For this review, use the dimensioned drawing (mm, ordinates from the lowest corner) and the shaded views. A direction names the side the tool comes from. Round coordinates to 2 decimals unless told otherwise and drop trailing zeros. Loops run counter-clockwise (first coordinate to the right, second up) from the corner with the lowest first, then second, coordinate; pieces in that order, holes last. Notation, with made-up numbers: (51.25, 47) - (74.25, 47) arc R10 cw to (74.25, 53) - close; hole circle Ø11 at (-40, -15). An arc over 180 degrees is marked (long way). Use one line per item in the form item = value. Start each with the question number.
(1) We need section B-B, the plane y = 5.25. Write out the cut boundary in (x, z).
(2) Machinability: for the marked faces 4, 5 and 6, which of the approach directions +Z, -Z, +X, -X, +Y, -Y give a long, thin tool a straight path to every point of the face, cutting with its end or side? Answer none if there is none.
(3) The part is to be moulded in two halves that separate along Z. For the marked faces 1, 2 and 3, say which applies: released by +Z, released by -Z, zero draft, split by the parting line, or undercut.
(4) Wall thickness on probe 1 along X at (y, z) = (0.75, 4.5); probe 2 along Z at (x, y) = (5.75, 3.25); probe 3 along Z at (x, y) = (3.75, 1): over which ranges is each line inside the solid? List them lowest first. Write a range as [from, to].
(5) We need section A-A, the plane x = 5.25. Write out the cut boundary in (y, z).
(6) For pin 1 (1.5 mm diameter, centred on x = 4.5, y = 2, fed in from -Z); pin 2 (1.5 mm diameter, centred on x = 4.5, z = 1.5, fed in from +Y), all flat-tipped, find the tip position at first contact; note any pin that passes through.
(7) We need section C-C, the plane x = 9.25. Write out the cut boundary in (y, z), then the cut area to 3 significant figures.
(8) We need section D-D, the plane z = 2. Write out the cut boundary in (x, y).
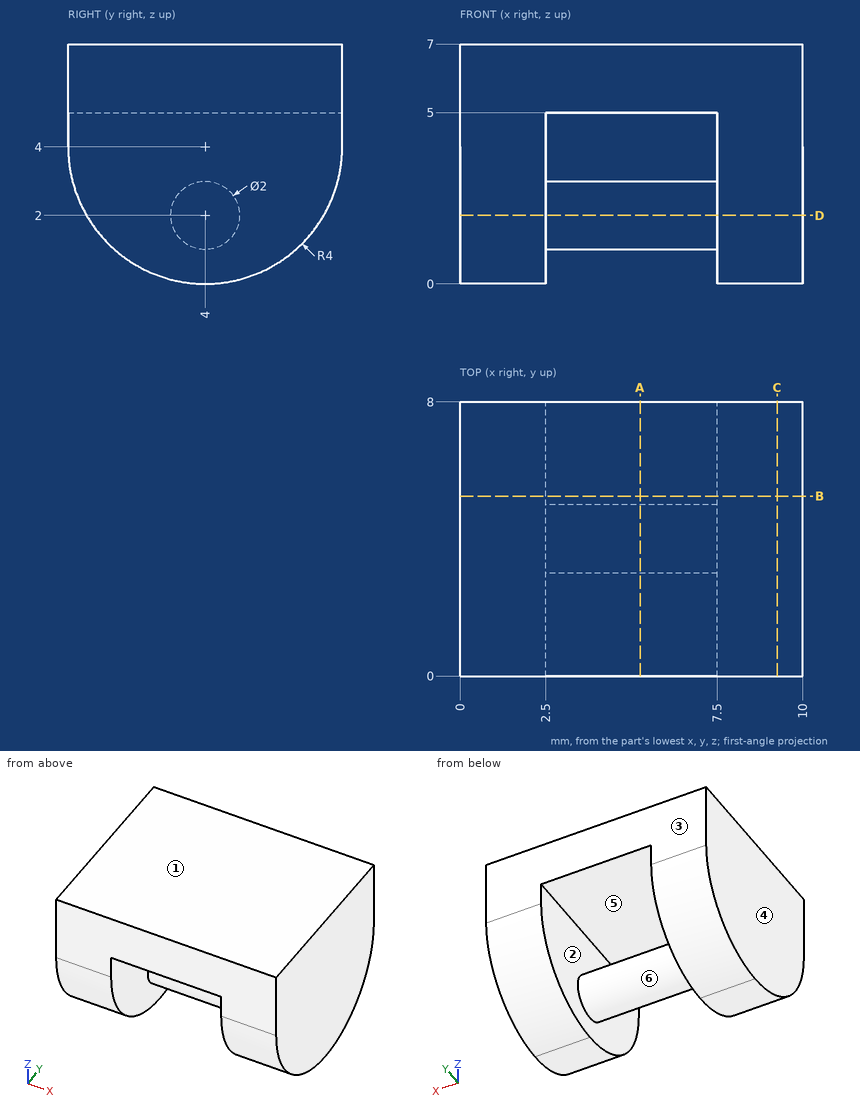
Data:
q1.outline = (0, 0.2) - (2.5, 0.2) - (2.5, 5) - (7.5, 5) - (7.5, 0.2) - (10, 0.2) - (10, 7) - (0, 7) - close
q2.face_4 = +Z, -Z, -X, +Y, -Y
q2.face_5 = +Y, -Y
q2.face_6 = none
q3.face_1 = released by +Z
q3.face_2 = undercut
q3.face_3 = zero draft
q4.probe_1 = [0, 2.5], [7.5, 10]
q4.probe_2 = [1.34, 2.66], [5, 7]
q4.probe_3 = [5, 7]
q5.outline = (0, 5) - (8, 5) - (8, 7) - (0, 7) - close; circle Ø2 at (4, 2)
q6.pin_1 = 5
q6.pin_2 = 5
q7.outline = (0, 4) arc R4 ccw to (8, 4) - (8, 7) - (0, 7) - close
q7.area = 49.1 mm^2
q8.outline = (0, 0.54) - (2.5, 0.54) - (2.5, 3) - (7.5, 3) - (7.5, 0.54) - (10, 0.54) - (10, 7.46) - (7.5, 7.46) - (7.5, 5) - (2.5, 5) - (2.5, 7.46) - (0, 7.46) - close
